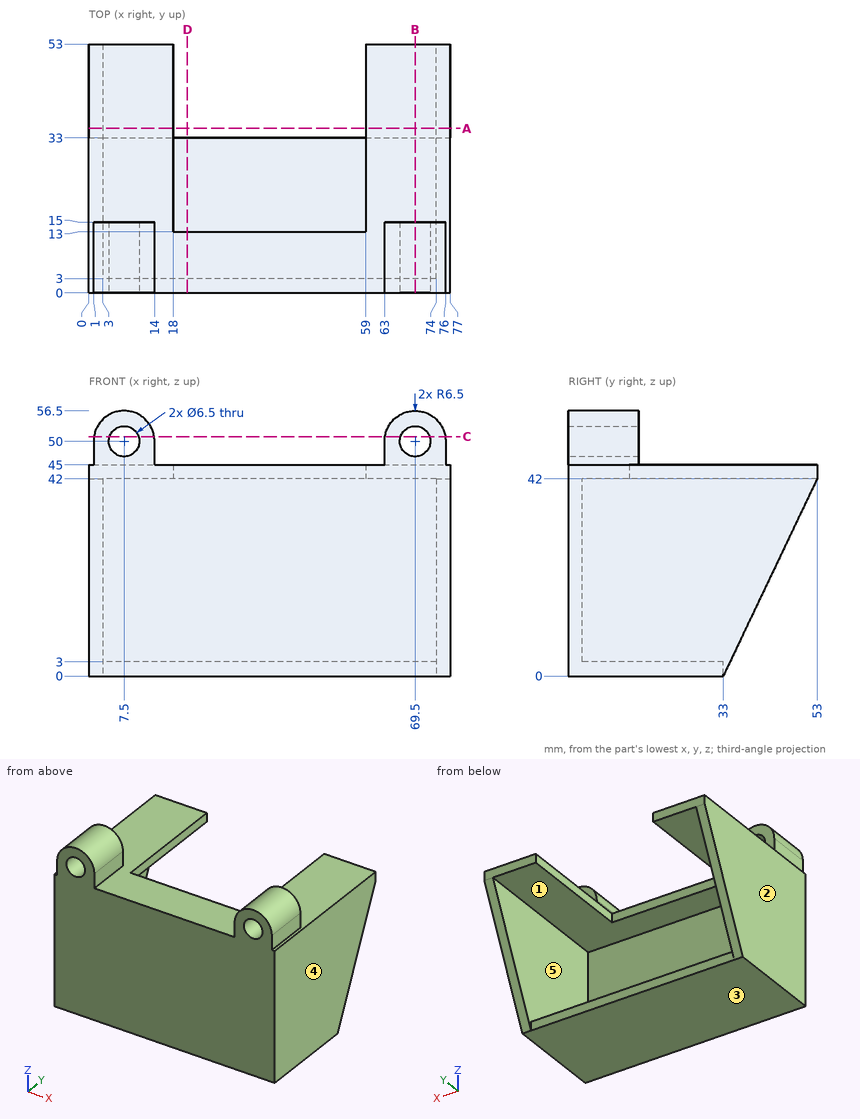
Geometry: see drawing. Coordinates: mm, zero at the bounding-box minimum. A direction names the side the tool comes from. Give positions to 0.01 mm unless a question says otherwise; leave off trailing zeros. Loops run counter-clockwise (first coordinate to the right, second up) from the corner with the lowest first, then second, coordinate; pieces in that order, holes last. Notation, with made-up numbers: (89, 56.5) -> (138, 56.5) arc R18 cw to (138, 66.5) -> close; hole circle Ø11 at (42.5, 8.5). An arc over 180 degrees is marked (long way). Put each result on its own line as item: value.
1. Set-up query: the marked faces 4 and 5. Return all of +Z, -Z, +X, -X, +Y, -Y with unobstructed straight access to the full face (end or side cutting, diameter ignored); none if empty.
Taken from the geometry:
face 4: +Z, -Z, +X, +Y, -Y
face 5: +Y
2. Pin query (flat end, axial travel): P1, Ø9, axis at x = 70, z = 51, coming from the +Y side; P2, Ø2.5, axis at x = 28.5, z = 44, coming from the +Y side; P3, Ø1, axis at x = 61, z = 16.5, coming from the +Y side; P4, Ø2, axis at x = 56.5, y = 43.5, coming from the -Z side. Return the tip coordinate at first contact, or that it passes through.
Taken from the geometry:
P1: stops at y = 15
P2: stops at y = 13
P3: stops at y = 3
P4: passes through
3. Cut plane C-C (z = 51). Return the cut outline in (x, y), plus the area to 3 significant figures.
Taken from the geometry:
outline: (1.08, 0) -> (4.41, 0) -> (4.41, 15) -> (1.08, 15) -> close; (10.59, 0) -> (13.92, 0) -> (13.92, 15) -> (10.59, 15) -> close; (63.08, 0) -> (66.41, 0) -> (66.41, 15) -> (63.08, 15) -> close; (72.59, 0) -> (75.92, 0) -> (75.92, 15) -> (72.59, 15) -> close
area: 200 mm2
4. Pull-direction query (X, two-part tool) for the marked faces 1, 2 and 3; classes: released by +X, released by -X, zero draft, split by the parting line, or undercut.
Taken from the geometry:
face 1: undercut
face 2: released by -X
face 3: zero draft
5. Cut plane B-B (x = 69.5). Return the cut outline in (y, z), plus the area to 3 significant figures.
Taken from the geometry:
outline: (0, 0) -> (33, 0) -> (33, 3) -> (3, 3) -> (3, 42) -> (53, 42) -> (53, 45) -> (15, 45) -> (15, 46.75) -> (0, 46.75) -> close; (0, 53.25) -> (15, 53.25) -> (15, 56.5) -> (0, 56.5) -> close
area: 450 mm2
6. Ray query, line 1 along X through (y, z) = (13.5, 11); line 2 along X through (y, z) = (9, 46.5); line 3 along Z through (x, y) = (25, 12). Return the intervals inside material, ascending. Write a range as [from, to].
Taken from the geometry:
line 1: x = [0, 3], [74, 77]
line 2: x = [1, 14], [63, 76]
line 3: z = [0, 3], [42, 45]
7. Cut plane D-D (x = 21). Return the cut outline in (y, z), plus the area to 3 significant figures.
Taken from the geometry:
outline: (0, 0) -> (33, 0) -> (33, 3) -> (3, 3) -> (3, 42) -> (13, 42) -> (13, 45) -> (0, 45) -> close
area: 255 mm2
8. Cut plane A-A (y = 35). Return the cut outline in (x, z).
Taken from the geometry:
outline: (0, 4.2) -> (3, 4.2) -> (3, 42) -> (18, 42) -> (18, 45) -> (0, 45) -> close; (59, 42) -> (74, 42) -> (74, 4.2) -> (77, 4.2) -> (77, 45) -> (59, 45) -> close
